Source: CAD feature listing. Evaluate the final solid. Frame: model axes, mm. A direction names the side the tool comes from. Give positions to 0.01 mm unless a question says otherwise; leave off trailing zeros. Write each loop counter-clockwise with the first axis right and the second up, starting at its lowest first coordinate (ties: lowest second). Pieces come first, ordered by that corner, then holes. Notation, with made-up numbers: M 56.25,-39.5 L 93.25,-39.5 A20 ccw 93.25,-10.5 Z; hole C 76.25,-25.75 d3. An arc over 180 degrees is marked long. Return JSON: item names as keys, results as strings.
```python
from build123d import *

# Parameters (mm, degrees)
F0_W      = 23
F0_H      = 20
F1_DEPTH  = 10
F3_DEPTH  = 15
F4_W      = 11
F4_H      = 3.5
F5_DEPTH  = 10.001
F6_DEPTH  = 3.5
F7_W      = 4.5
F7_H      = 15
F7_W_2    = 18.5
F8_DEPTH  = 3
F9_DEPTH  = 7
F10_R     = 2.5
F11_DEPTH = 10.001
F10_R_2   = 5
F12_DEPTH = 4.5
F16_R     = 1.15
F17_DEPTH = 10
F18_R     = 2.25
F19_DEPTH = 10.001
F20_DEPTH = 5
F21_DEPTH = 10.001
F22_W     = 2.5
F22_H     = 2.5
F23_DEPTH = 10.001
F24_W     = 9
F24_H     = 9
F25_DEPTH = 15.751
F26_W     = 3.5
F26_H     = 9
F27_DEPTH = 23.001


# Not quite as in the source:
# - a feature names something its author has since deleted; it is built from what else it names


with BuildPart() as f1:
    # F0 (on Top) → F1 (new body)
    with BuildSketch(Plane.XY):
        Rectangle(F0_W, F0_H)
    extrude(amount=F1_DEPTH)

    # F2 (on face) → F3 (join)
    with BuildSketch(Plane.XY.offset(10)):
        Polygon((5.5, -6.5), (5.5, -10), (11.5, -10), (11.5, -0.75), (7, -0.75), (7, -4.25), (8.25, -4.25), (8.25, -6.5), align=None)
        Polygon((-11.5, -10), (-5.5, -10), (-5.5, -6.5), (-8.25, -6.5), (-8.25, -4.25), (-7, -4.25), (-7, -0.75), (-11.5, -0.75), align=None)
    extrude(amount=F3_DEPTH)

    # F4 (on face) → F5 (cut, through all)
    with BuildSketch(Plane.XY.offset(10)):
        with Locations((0, -8.25)):
            Rectangle(F4_W, F4_H)
    extrude(amount=-F5_DEPTH, mode=Mode.SUBTRACT)

    # F6 (add): faces of the model
    f6_faces = [f1.faces().sort_by_distance(p)[0] for p in [
        (9.25, -0.75, 17.5),
        (-9.25, -0.75, 17.5),
    ]]
    extrude(f6_faces, amount=F6_DEPTH)

    # F7 (on face) → F8 (join)
    with BuildSketch(Plane(origin=(0, 2.75, 0), x_dir=(-1, 0, 0), z_dir=(0, 1, 0))):
        with Locations((-9.25, 17.5)):
            Rectangle(F7_W, F7_H)
        with Locations((2.25, 17.5)):
            Rectangle(F7_W_2, F7_H)
    extrude(amount=F8_DEPTH)

    # F9 (add): a face of the model
    f9_faces = [f1.faces().sort_by_distance(p)[0] for p in [
        (0, 10, 5),
    ]]
    extrude(f9_faces, amount=F9_DEPTH)

    # F10 (on face) → F11 (cut, through all)
    with BuildSketch(Plane.XY.offset(10)):
        with Locations((0, 11.25)):
            Circle(F10_R)
    extrude(amount=-F11_DEPTH, mode=Mode.SUBTRACT)

    # F10 (on face) → F12 (cut)
    with BuildSketch(Plane.XY.offset(10)):
        with Locations((0, 11.25)):
            Circle(F10_R_2)
        with Locations((0, 11.25)):
            Circle(F10_R, mode=Mode.SUBTRACT)
    extrude(amount=-F12_DEPTH, mode=Mode.SUBTRACT)

    # F16 (on face) → F17 (cut)
    with BuildSketch(Plane.XY.offset(25)):
        with Locations((-9, -2.125)):
            Circle(F16_R)
        with Locations((9, -2.125)):
            Circle(F16_R)
    extrude(amount=-F17_DEPTH, mode=Mode.SUBTRACT)

    # F18 (on face) → F19 (cut, through all)
    with BuildSketch(Plane.XY.offset(10)):
        with Locations((0, -1.5)):
            Circle(F18_R)
    extrude(amount=-F19_DEPTH, mode=Mode.SUBTRACT)

    # F18 (on face) → F20 (cut)
    with BuildSketch(Plane.XY.offset(10)):
        with BuildLine():
            ThreePointArc((0, 2.75), (-3.00520382, -4.50520382), (4.25, -1.5))
            ThreePointArc((4.25, -1.5), (3.00520382, 1.50520382), (0, 2.75))
        make_face()
        with Locations((0, -1.5)):
            Circle(F18_R, mode=Mode.SUBTRACT)
    extrude(amount=-F20_DEPTH, mode=Mode.SUBTRACT)

    # F21 (cut, through all): faces of the model
    f21_faces = [f1.faces().sort_by_distance(p)[0] for p in [
        (-11.2439604523, 11.375, 10),
        (-4.8585786438, 11.25, 5.5),
    ]]
    extrude(f21_faces, amount=-F21_DEPTH, mode=Mode.SUBTRACT)

    # F22 (on face) → F23 (cut, through all)
    with BuildSketch(Plane.XY.offset(10)):
        with Locations((5.75, 1.5)):
            Rectangle(F22_W, F22_H)
    extrude(amount=-F23_DEPTH, mode=Mode.SUBTRACT)

    # F24 (on face) → F25 (cut, through all)
    with BuildSketch(Plane(origin=(0, 5.75, 0), x_dir=(-1, 0, 0), z_dir=(0, 1, 0))):
        with Locations((0, 15)):
            Rectangle(F24_W, F24_H)
    extrude(amount=-F25_DEPTH, mode=Mode.SUBTRACT)

    # F26 (on face) → F27 (cut, through all)
    with BuildSketch(Plane.YZ.offset(11.5)):
        with Locations((-8.25, 15)):
            Rectangle(F26_W, F26_H)
    extrude(amount=-F27_DEPTH, mode=Mode.SUBTRACT)


solid = f1.part
```
1) Cut plane C-C, the plane z = 8. Return the cut outline in (x, y), then the cut area to 3 significant figures.
Numbers:
{"outline": "M -11.5,-10 L -5.5,-10 L -5.5,-6.5 L 5.5,-6.5 L 5.5,-10 L 11.5,-10 L 11.5,5.75 L -11.5,5.75 Z; hole C 0,-1.5 d8.5; hole M 4.5,0.25 L 7,0.25 L 7,2.75 L 4.5,2.75 Z", "area": "261 mm²"}
2) Contact query for flat-ended pins moving along their axis: pin 1 Ø6 at (x, y) = (0, -1.5) entering from +Z; pin 2 Ø5 at (x, z) = (0, 4) entering from -Y; pin 3 Ø2 at (x, y) = (-9, -2.125) entering from +Z. Output: stop coordinate, or through.
Numbers:
{"pin 1": "stops at z = 5", "pin 2": "stops at y = -6.5", "pin 3": "stops at z = 15"}
3) Line query: line 1 (X direction, y = -1.25, z = 9.75); line 2 (X direction, y = 2, z = 3.5); line 3 (Z direction, x = -10.25, y = -9). Output: solid intervals per line, ascending. Write a range as [from, to].
Numbers:
{"line 1": "x = [-11.5, -4.24], [4.24, 11.5]", "line 2": "x = [-11.5, 4.5], [7, 11.5]", "line 3": "z = [0, 10.5], [19.5, 25]"}
4) Set-up query: faces 4 (the face through (10, -6.5, 15)), 5 (the face through (6, 0.25, 5)), 6 (the face through (0, 4, 19.5)), 7 (the face through (5, 2.75, 15)). Return all of +Z, -Z, +X, -X, +Y, -Y with unobstructed straight access to the full face (end or side cutting, diameter ignored); none if empty.
Numbers:
{"face 4": "+X, -X, -Y", "face 5": "+Z, -Z", "face 6": "+Y, -Y", "face 7": "+Z"}
5) Cut plane A-A, the plane x = -3.75. Return the cut outline in (y, z).
Numbers:
{"outline": "M -6.5,0 L 5.75,0 L 5.75,10.5 L 2.75,10.5 L 2.75,10 L 0.5,10 L 0.5,5 L -3.5,5 L -3.5,10 L -6.5,10 Z; M 2.75,19.5 L 5.75,19.5 L 5.75,25 L 2.75,25 Z"}
6) Draft query along X for faces 1 (the face through (-5.5, -8, 22)), 2 (the face through (-9, -10, 5)), 3 (the face through (-11.5, -2, 12)). Return one class per face: released by +X, released by -X, zero draft, split by the parting line, or undercut.
Numbers:
{"face 1": "undercut", "face 2": "zero draft", "face 3": "released by -X"}
7) Cut plane B-B, the plane z = 17. Return the cut outline in (x, y) (3 decimals), then the cut area to 3 significant figures.
Numbers:
{"outline": "M -11.5,-6.5 L -8.25,-6.5 L -8.25,-4.25 L -7,-4.25 L -7,2.75 L -4.5,2.75 L -4.5,5.75 L -11.5,5.75 Z; M 4.5,2.75 L 7,2.75 L 7,-4.25 L 8.25,-4.25 L 8.25,-6.5 L 11.5,-6.5 L 11.5,5.75 L 4.5,5.75 Z; hole C -9,-2.125 d2.3; hole C 9,-2.125 d2.3", "area": "111 mm²"}
8) Cut plane D-D, the plane x = 1.25. Return the cut outline in (y, z).
Numbers:
{"outline": "M -6.5,0 L -3.37,0 L -3.37,5 L -5.56,5 L -5.56,10 L -6.5,10 Z; M 0.37,0 L 5.75,0 L 5.75,10.5 L 2.75,10.5 L 2.75,10 L 2.56,10 L 2.56,5 L 0.37,5 Z; M 2.75,19.5 L 5.75,19.5 L 5.75,25 L 2.75,25 Z"}
